Verification items for this drawing (mm, ordinates from the low corner). Give positions to 0.01 mm unless a question says otherwise; leave off trailing zeros. Loops run counter-clockwise (first coordinate to the right, second up) from the corner with the lowest first, then second, coordinate; pieces in that order, holes last. Notation, with made-up numbers: (-6, 42) -> (0, 42) arc R9 cw to (0, 54) -> close; hole circle Ø11 at (85.25, 18.5). An arc over 180 degrees is marked (long way). Write each question's results on one line, items separated by ' | '. Start each with the question number.
1) Sectioned sample at B-B on y = 0.7. Record the cut outline in (x, z).
2) Sectioned sample at A-A on x = 5.75. Record the cut outline in (y, z).
3) Scan lines: line 1 (Z direction, x = 13, y = 0.45); line 2 (Z direction, x = 12.5, y = 0.8). Record each from-to range of solid material in increasing order. Write a range as from..to.
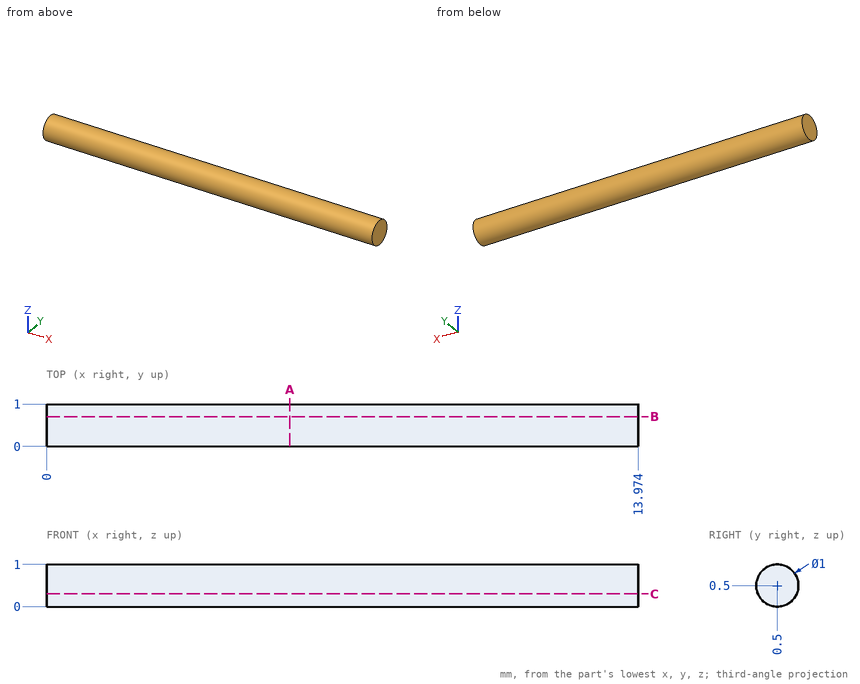
Result:
1) outline: (0, 0.04) -> (13.97, 0.04) -> (13.97, 0.96) -> (0, 0.96) -> close
2) outline: circle Ø1 at (0.5, 0.5)
3) line 1: 0..1 | line 2: 0.1..0.9
